Part print with two shaded views. Sizes in mm from the minimum x, y, z corner. A direction names the side the tool comes from. Round coordinates to 2 decimals unless told otherwise and drop trailing zeros. Loops run counter-clockwise (first coordinate to the right, second up) from the corner with the lowest first, then second, coordinate; pieces in that order, holes last. Notation, with made-up numbers: (58, 68) -> (91, 68) arc R15 ccw to (91, 94) -> close; hole circle Ø2 at (-38, -4). An arc over 180 degrees is marked (long way). Put each result on its own line as item: value. Start each with the question number.
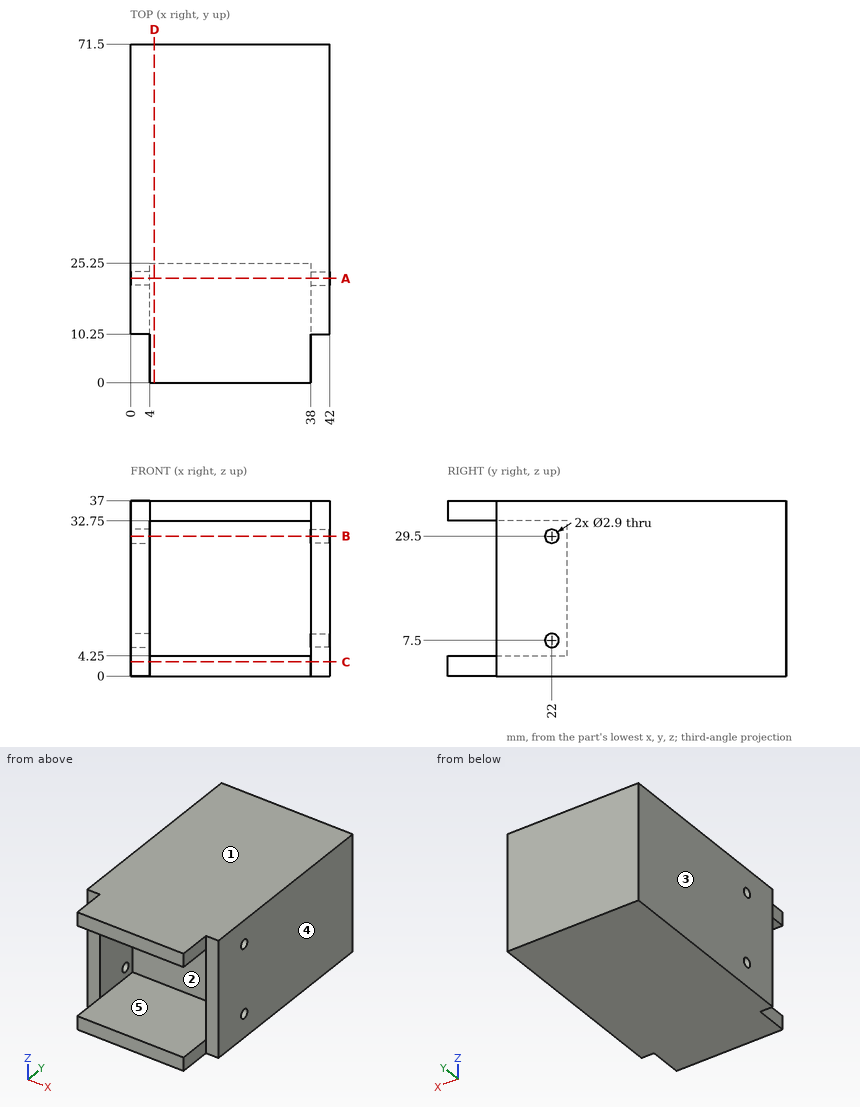
Item 1: 3-axis set-ups, long thin cutter, end or side, ignore diameter. For the marked faces 4 and 5: which of +Z, -Z, +X, -X, +Y, -Y reach the whole face in a straight line?
Item 2: Drop flat-ended pins along their axis: pin 1 (4.5 mm diameter, centred on y = 6, z = 3, fed in from -X); pin 2 (1.5 mm diameter, centred on x = 19.5, y = 31, fed in from -Z); pin 3 (2 mm diameter, centred on x = 2, z = 24.5, fed in from -Y); pin 4 (3.5 mm diameter, centred on y = 7.5, z = 35.5, fed in from +X). Give the stop position or say it passes through.
Item 3: Cut at B-B on z = 29.5. Write the cut outline in (x, y).
Item 4: Cut at A-A on y = 22. Write the cut outline in (x, z), then the cut area to 3 significant figures.
Item 5: Wall check: line 1 (Z direction, x = 3, y = 22); line 2 (Y direction, x = 41.15, z = 7.5); line 3 (X direction, y = 13, z = 19). Give the ranges that are in metal, low to high. Write a range as from..to.
Item 6: Pull direction X, two halves, no side cores. Call the marked faces 1, 2 and 3: +X half, -X half, draft (parallel to the pull), parting line (faces both ways), or undercut.
Item 7: Cut at C-C on z = 3. Write the cut outline in (x, y).
Item 8: Cut at D-D on x = 5. Write the cut outline in (y, z).
Ans:
1. face 4: +Z, -Z, +X, +Y, -Y
1. face 5: -Y
2. pin 1: stops at x = 4
2. pin 2: stops at z = 0
2. pin 3: stops at y = 10.25
2. pin 4: stops at x = 38
3. outline: (0, 10.25) -> (4, 10.25) -> (4, 20.55) -> (0, 20.55) -> close; (0, 23.45) -> (4, 23.45) -> (4, 25.25) -> (38, 25.25) -> (38, 23.45) -> (42, 23.45) -> (42, 71.5) -> (0, 71.5) -> close; (38, 10.25) -> (42, 10.25) -> (42, 20.55) -> (38, 20.55) -> close
4. outline: (0, 0) -> (42, 0) -> (42, 6.05) -> (38, 6.05) -> (38, 4.25) -> (4, 4.25) -> (4, 6.05) -> (0, 6.05) -> close; (0, 8.95) -> (4, 8.95) -> (4, 28.05) -> (0, 28.05) -> close; (0, 30.95) -> (4, 30.95) -> (4, 32.75) -> (38, 32.75) -> (38, 30.95) -> (42, 30.95) -> (42, 37) -> (0, 37) -> close; (38, 8.95) -> (42, 8.95) -> (42, 28.05) -> (38, 28.05) -> close
4. area: 539 mm2
5. line 1: z = 0..6.05, 8.95..28.05, 30.95..37
5. line 2: y = 10.25..20.55, 23.45..71.5
5. line 3: x = 0..4, 38..42
6. face 1: draft
6. face 2: undercut
6. face 3: -X half
7. outline: (0, 10.25) -> (4, 10.25) -> (4, 0) -> (38, 0) -> (38, 10.25) -> (42, 10.25) -> (42, 71.5) -> (0, 71.5) -> close
8. outline: (0, 0) -> (71.5, 0) -> (71.5, 37) -> (0, 37) -> (0, 32.75) -> (25.25, 32.75) -> (25.25, 4.25) -> (0, 4.25) -> close
